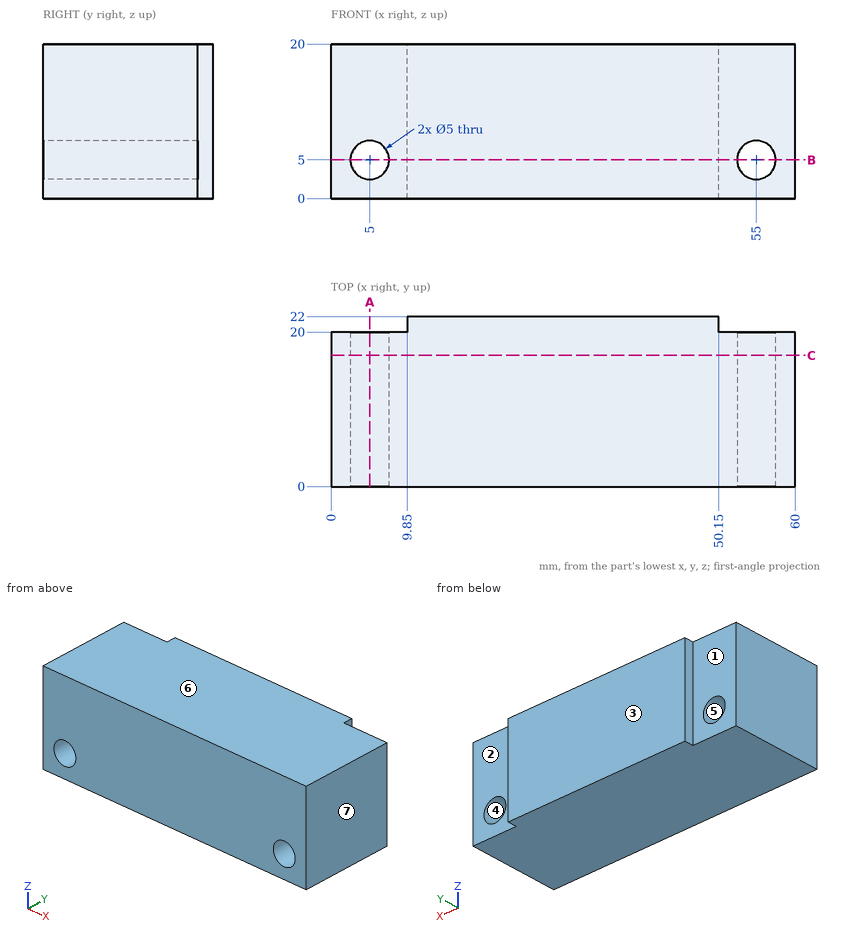
Print and shaded views of the part. All mm, measured from the part's lowest x, y and z. A direction names the side the tool comes from. Round coordinates to 2 decimals unless told otherwise and drop trailing zeros. Write each loop counter-clockwise with the first axis right and the second up, starting at its lowest first coordinate (ties: lowest second). Pieces come first, ordered by that corner, then holes. Notation, with made-up numbers: (8, 70.5) -> (16, 70.5) arc R25 ccw to (16, 83.5) -> close; hole circle Ø3 at (79.25, 37.25). An arc over 180 degrees is marked (long way). Return JSON: item names as keys, results as strings. Group by question number.
Q1. Which spindle directions (+Z, -Z, +X, -X, +Y, -Y) get a long thin tool onto all of the face, cutting with end or side? Do the marked faces 1, 2 and 3. Say none if no direction does.
Q2. Saw through at A-A on x = 5. Write the cut outline in (y, z).
Q3. Saw through at B-B on z = 5. Write the cut outline in (x, y).
Q4. Mould opens along Z. For the marked faces 4, 5, 6 and 7 say: pulls with the +Z half, pulls with the -Z half, needs draft (parallel to the pull), parting line crosses it, or undercut.
Q5. Probe L1, parallel to Z at x = 5, y = 11; L2, parallel to X at y = 13.25, z = 6; L3, parallel to Z at x = 56, y = 19.75. List the from-to ranges inside material, lowest first. Write a range as [from, to].
Q6. Pin check, flat tip, straight feed: pin 1 (0.6 mm diameter, centred on y = 20.5, z = 6.5, fed in from -X). Stop position of the tip, or through.
Q7. Saw through at C-C on y = 17. Write the cut outline in (x, z).
Answer:
{
 "1": {"face 1": "+Z, -Z, -X, +Y", "face 2": "+Z, -Z, +X, +Y", "face 3": "+Z, -Z, +X, -X, +Y"},
 "2": {"outline": "(0, 0) -> (20, 0) -> (20, 2.5) -> (0, 2.5) -> close; (0, 7.5) -> (20, 7.5) -> (20, 20) -> (0, 20) -> close"},
 "3": {"outline": "(0, 0) -> (2.5, 0) -> (2.5, 20) -> (0, 20) -> close; (7.5, 0) -> (52.5, 0) -> (52.5, 20) -> (50.15, 20) -> (50.15, 22) -> (9.85, 22) -> (9.85, 20) -> (7.5, 20) -> close; (57.5, 0) -> (60, 0) -> (60, 20) -> (57.5, 20) -> close"},
 "4": {"face 4": "undercut", "face 5": "undercut", "face 6": "pulls with the +Z half", "face 7": "needs draft"},
 "5": {"L1": "[0, 2.5], [7.5, 20]", "L2": "[0, 2.71], [7.29, 52.71], [57.29, 60]", "L3": "[0, 2.71], [7.29, 20]"},
 "6": {"pin 1": "x = 9.85"},
 "7": {"outline": "(0, 0) -> (60, 0) -> (60, 20) -> (0, 20) -> close; hole circle Ø5 at (5, 5); hole circle Ø5 at (55, 5)"}
}
